Verification items for the finished model (mm, model axes). Face numbers are marked on the shaded views. Round coordinates to 2 decimals unless told otherwise and drop trailing zeros. Write each loop counter-clockwise with the first axis right and the second up, starting at its lowest first coordinate (ties: lowest second). Pieces come first, ordered by that corner, then holes. Notation, with made-up numbers: M 29.5,-27 L 62.5,-27 A24 cw 62.5,7 Z; hole C -23,10 d3. An arc over 180 degrees is marked long. One line per item, written item: value. Start each with the question number.
from build123d import *

# Parameters (mm, degrees)
SKETCH1_R           = 26.67
BOSS_EXTRUDE1_DEPTH = 81.28
SHELL1_T            = -2.54
SKETCH2_R           = 26.67
SKETCH2_R_2         = 15.875
BOSS_EXTRUDE2_DEPTH = 3.81


with BuildPart() as part:
    # Sketch1 → Boss-Extrude1 (new body)
    with BuildSketch(Plane(origin=(0, 0, 0), x_dir=(1, 0, 0), z_dir=(0, 1, 0))):
        with Locations(Location((0, 0, 0), (0, 0, 270))):
            Circle(SKETCH1_R)
    extrude(amount=BOSS_EXTRUDE1_DEPTH)

    # Shell1
    shell1_openings = [part.faces().sort_by_distance(p)[0] for p in [
        (0, 81.28, 0),
    ]]
    offset(amount=SHELL1_T, openings=shell1_openings, kind=Kind.INTERSECTION)

    # Sketch2 → Boss-Extrude2 (add)
    with BuildSketch(Plane(origin=(0, 81.28, 0), x_dir=(1, 0, 0), z_dir=(0, 1, 0))):
        with Locations(Location((0, 0, 0), (0, 0, 270))):
            Circle(SKETCH2_R)
        with Locations(Location((0, 0, 0), (0, 0, 90))):
            Circle(SKETCH2_R_2, mode=Mode.SUBTRACT)
    extrude(amount=BOSS_EXTRUDE2_DEPTH)


solid = part.part
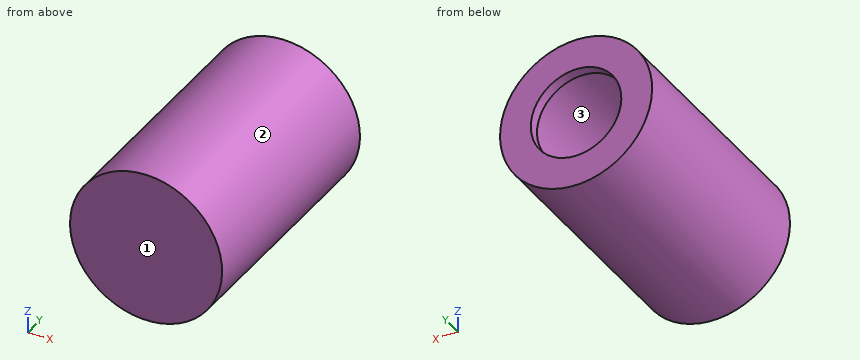
1) Cross-section at A-A (z = 0). Record the boundary of the cut face in (x, y) (3 decimals), then the cut area to 3 significant figures.
2) Cross-section at B-B (x = 0). Record the boundary of the cut face in (y, z) (3 decimals).
3) Gauge pin test, flat ends, axial feed: pin 1 Ø6 at (x, y) = (-18, 47.5) entering from -Z; pin 2 Ø4 at (y, z) = (69, 10.5) entering from +X; pin 3 Ø5 at (x, z) = (-11, -1) entering from +Y. Record the tip position at first contact, or that the pin passes through.
4) Cross-section at D-D (y = 37). Record the boundary of the cut face in (x, z), then the cut area to 3 significant figures.
5) Thickness scan on line 1 (Y direction, x = -12, z = -17.5); line 2 (X direction, y = 83, z = 0) (3 decimals); line 3 (Z direction, x = -1, y = 52). Record the ranges inside material, lowest first.
6) Mould release check, pull along X, two halves, no side actions. Record for the marked faces 1, 2 and 3: pulls with the +X half, pulls with the -X half, needs draft (parallel to the pull), parting line crosses it, or undercut.
7) Cross-section at C-C (z = 17.5). Record the boundary of the cut face in (x, y), then the cut area to 3 significant figures.
Results below:
1. outline: M -26.67,0 L 26.67,0 L 26.67,85.09 L 15.875,85.09 L 15.875,81.28 L 24.13,81.28 L 24.13,2.54 L -24.13,2.54 L -24.13,81.28 L -15.875,81.28 L -15.875,85.09 L -26.67,85.09 Z
1. area: 618 mm²
2. outline: M 0,-26.67 L 85.09,-26.67 L 85.09,-15.875 L 81.28,-15.875 L 81.28,-24.13 L 2.54,-24.13 L 2.54,24.13 L 81.28,24.13 L 81.28,15.875 L 85.09,15.875 L 85.09,26.67 L 0,26.67 Z
3. pin 1: stops at z = -22.05
3. pin 2: stops at x = 25.28
3. pin 3: stops at y = 2.54
4. outline: C 0,0 d53.34; hole C 0,0 d48.26
4. area: 405 mm²
5. line 1: y = 0 to 2.54, 81.28 to 85.09
5. line 2: x = -26.67 to -15.875, 15.875 to 26.67
5. line 3: z = -26.65 to -24.11, 24.11 to 26.65
6. face 1: needs draft
6. face 2: parting line crosses it
6. face 3: undercut
7. outline: M -20.13,0 L 20.13,0 L 20.13,85.09 L -20.13,85.09 Z; hole M -16.61,2.54 L 16.61,2.54 L 16.61,81.28 L -16.61,81.28 Z
7. area: 809 mm²
